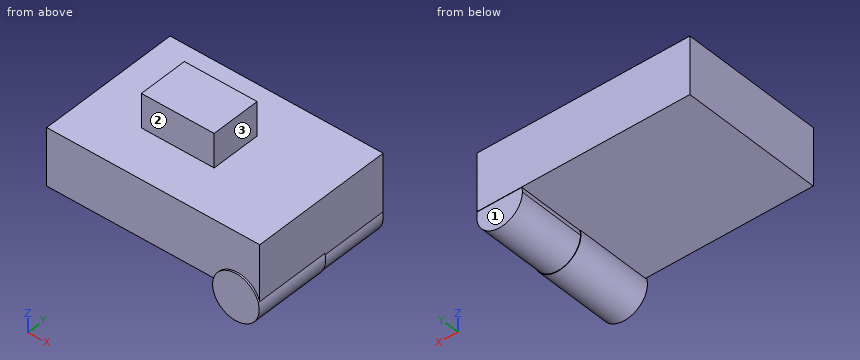
```python
from build123d import *

# Parameters (mm, degrees)
F0_W     = 93.85059
F0_H     = 63.135851
F1_DEPTH = 25.4
F2_R     = 10.276796
F3_DEPTH = 34.036
F5_DEPTH = 29.718
F6_W     = 32.04192
F6_H     = 21.99327
F7_DEPTH = 14.986


with BuildPart() as f1:
    # F0 (on Top) → F1 (new body)
    with BuildSketch(Plane.XY):
        with Locations((9.290259, -1.706374)):
            Rectangle(F0_W, F0_H)
    extrude(amount=F1_DEPTH)

    # F2 (on Front) → F3 (join)
    with BuildSketch(Plane.XZ):
        with Locations((46.356503, -2.180367)):
            Circle(F2_R)
    extrude(amount=F3_DEPTH)

    # F4 (on face) → F5 (join)
    with BuildSketch(Plane(origin=(0, 0, 0), x_dir=(-1, 0, 0), z_dir=(0, 1, 0))):
        with BuildLine():
            ThreePointArc((-56.173078, 0), (-47.453229, -12.176184), (-36.300701, -2.180367))
            ThreePointArc((-36.300701, -2.180367), (-36.360687, -1.083641), (-36.539928, 0))
            Line((-36.539928, 0), (-56.173078, 0))
        make_face()
    extrude(amount=F5_DEPTH)

    # F6 (on face) → F7 (join)
    with BuildSketch(Plane.XY.offset(25.4)):
        with Locations((2.464763, -1.801173)):
            Rectangle(F6_W, F6_H)
    extrude(amount=F7_DEPTH)


solid = f1.part
```
Check sheet for the modelled part. Datum: model origin and axes. Units: mm. Face numbers are marked on the shaded views. A direction names the side the tool comes from. Give positions to 0.01 mm unless a question says otherwise; leave off trailing zeros. Order: outer loops, then holes, each group sorted by start corner. A loop starts at its lowest first (then second) coordinate and runs counter-clockwise, first axis right, second up. Notation, with made-up numbers: M -3,63.5 L 33,63.5 A27 ccw 33,81.5 Z; hole C 12,72 d4. An arc over 180 degrees is marked long. Answer in a Markdown table with one row per item. Add a question column.
Q1. Access from +Z, -Z, +X, -X, +Y, -Y to the whole of each face (thin tool, end or side, straight path). Record for the marked faces 1, 2 and 3.
Q2. Thickness scan on L1, parallel to Z at x = 47, y = -11.5; L2, parallel to X at y = -7, z = 30; L3, parallel to Z at x = 13.5, y = -31. Record the ranges inside material, lowest first.
Q3. Sectioned sample at B-B, the plane y = 8. Record the boundary of the cut face in (x, z), and give its area (3 significant figures).
Q4. Gauge pin test, flat ends, axial feed: pin 1 Ø7.5 at (x, z) = (-3, 31) entering from +Y; pin 2 Ø7.5 at (x, z) = (-5, 34) entering from -Y; pin 3 Ø8 at (y, z) = (-14.5, -6) entering from -X; pin 4 Ø10.5 at (x, z) = (43.5, -5) entering from +Y. Record the tip position at first contact, or that the pin passes through.
Q5. Sectioned sample at A-A, the plane x = -7.5. Record the boundary of the cut face in (y, z), and give its area (3 significant figures).
Q6. Sectioned sample at D-D, the plane y = 24. Record the boundary of the cut face in (x, z), and give its area (3 significant figures).
Q7. Sectioned sample at C-C, the plane z = -4. Record the boundary of the cut face in (x, y), and give its area (3 significant figures).
Verdict:
| question | item | result |
|---|---|---|
| 1 | face 1 | -Z, +X, -X, +Y |
| 1 | face 2 | +Z, +X, -X, -Y |
| 1 | face 3 | +Z, +X, +Y, -Y |
| 2 | L1 | -12.44 to 25.4 |
| 2 | L2 | -13.56 to 18.49 |
| 2 | L3 | 0 to 25.4 |
| 3 | outline | M -37.64,0 L 36.54,0 A10.06 ccw 36.3,-2.18 A10.06 ccw long 56.17,0 L 56.22,0 L 56.22,25.4 L 18.49,25.4 L 18.49,40.39 L -13.56,40.39 L -13.56,25.4 L -37.64,25.4 Z |
| 3 | area | 3,070 mm² |
| 4 | pin 1 | y = 9.2 |
| 4 | pin 2 | y = -12.8 |
| 4 | pin 3 | x = 36.08 |
| 4 | pin 4 | y = 29.86 |
| 5 | outline | M -33.27,0 L 29.86,0 L 29.86,25.4 L 9.2,25.4 L 9.2,40.39 L -12.8,40.39 L -12.8,25.4 L -33.27,25.4 Z |
| 5 | area | 1,930 mm² |
| 6 | outline | M -37.64,0 L 36.54,0 A10.06 ccw 36.3,-2.18 A10.06 ccw long 56.17,0 L 56.22,0 L 56.22,25.4 L -37.64,25.4 Z |
| 6 | area | 2,590 mm² |
| 7 | outline | M 36.24,-34.04 L 56.47,-34.04 L 56.47,0 L 56.25,0 L 56.25,29.72 L 36.47,29.72 L 36.47,0 L 36.24,0 Z |
| 7 | area | 1,280 mm² |
